Verification items for the finished model (mm, model axes). A direction names the side the tool comes from. Give positions to 0.01 mm unless a question says otherwise; leave off trailing zeros. Write each loop counter-clockwise with the first axis right and the second up, starting at its lowest first coordinate (ties: lowest second). Pieces come first, ordered by that corner, then holes.
from build123d import *

# Parameters (mm, degrees)
SKETCH_1_W             = 38
SKETCH_1_H             = 30
SKETCH_1_R             = 1.65
EXTRUDE_694_DEPTH      = 25
SKETCH_3_W             = 20
SKETCH_3_H             = 30
CUT_EXTRUDE_926_DEPTH  = 15
SKETCH_4_W             = 2.3
SKETCH_4_H             = 15
CUT_EXTRUDE_1406_DEPTH = 55.488530903
FILLET_3_R             = 1
FILLET_4_R             = 2
SKETCH_6_R             = 1.75
CUT_EXTRUDE_2902_DEPTH = 55.488530903
SKETCH_7_R             = 3.5
CUT_EXTRUDE_3145_DEPTH = 10
CUT_EXTRUDE_3527_DEPTH = 3


with BuildPart() as part:
    # Эскиз1 → Extrude 694 (new body)
    with BuildSketch(Plane(origin=(0, 0, 0), x_dir=(1, 0, 0), z_dir=(0, 1, 0))):
        with Locations((19, 15)):
            Rectangle(SKETCH_1_W, SKETCH_1_H)
        with Locations(Location((14.050252532, 24.949747468, 0), (0, 0, 270))):
            Circle(SKETCH_1_R, mode=Mode.SUBTRACT)
        with Locations(Location((23.949747468, 24.949747468, 0), (0, 0, 270))):
            Circle(SKETCH_1_R, mode=Mode.SUBTRACT)
        with Locations(Location((23.949747468, 15.050252532, 0), (0, 0, 270))):
            Circle(SKETCH_1_R, mode=Mode.SUBTRACT)
        with Locations(Location((14.050252532, 15.050252532, 0), (0, 0, 270))):
            Circle(SKETCH_1_R, mode=Mode.SUBTRACT)
    extrude(amount=EXTRUDE_694_DEPTH)

    # Эскиз3 → Cut-Extrude 926 (cut)
    with BuildSketch(Plane(origin=(0, 25, 0), x_dir=(1, 0, 0), z_dir=(0, 1, 0))):
        with Locations((19, 15)):
            Rectangle(SKETCH_3_W, SKETCH_3_H)
    extrude(amount=-CUT_EXTRUDE_926_DEPTH, mode=Mode.SUBTRACT)

    # Эскиз4 → Cut-Extrude 1406 (cut, through all)
    with BuildSketch(Plane.ZY):
        Polygon((-30, 10), (-23, 25), (-30, 25), align=None)
        with Locations((-9.900252532, 17.5)):
            Rectangle(SKETCH_4_W, SKETCH_4_H)
    extrude(amount=-CUT_EXTRUDE_1406_DEPTH, mode=Mode.SUBTRACT)

    # Скругление3
    fillet_3_edges = [part.edges().sort_by_distance(p)[0] for p in [
        (4.5, 25, -11.050252532),
        (33.5, 25, -11.050252532),
        (4.5, 25, -8.750252532),
        (33.5, 25, -8.750252532),
    ]]
    fillet(fillet_3_edges, radius=FILLET_3_R)

    # Скругление4
    fillet_4_edges = [part.edges().sort_by_distance(p)[0] for p in [
        (9, 17.5, 0),
        (19, 10, 0),
        (29, 17.5, 0),
        (38, 0, -15),
        (0, 0, -15),
        (9, 17.5, -26.5),
        (29, 17.5, -26.5),
        (38, 17.5, -26.5),
        (0, 17.5, -26.5),
    ]]
    fillet(fillet_4_edges, radius=FILLET_4_R)

    # Эскиз6 → Cut-Extrude 2902 (cut, through all)
    with BuildSketch(Plane(origin=(0, 0, -30), x_dir=(-1, 0, 0), z_dir=(0, 0, -1))):
        with Locations((-34, 15)):
            Circle(SKETCH_6_R)
        with Locations((-4, 15)):
            Circle(SKETCH_6_R)
    extrude(amount=-CUT_EXTRUDE_2902_DEPTH, mode=Mode.SUBTRACT)

    # Эскиз7 → Cut-Extrude 3145 (cut)
    with BuildSketch(Plane(origin=(0, 0, -30), x_dir=(-1, 0, 0), z_dir=(0, 0, -1))):
        with Locations((-34, 15)):
            Circle(SKETCH_7_R)
        with Locations((-4, 15)):
            Circle(SKETCH_7_R)
    extrude(amount=-CUT_EXTRUDE_3145_DEPTH, mode=Mode.SUBTRACT)

    # Эскиз8 → Cut-Extrude 3527 (cut)
    with BuildSketch(Plane.XY):
        Polygon((7, 13.267949192), (7, 16.732050808), (4, 18.464101615), (1, 16.732050808), (1, 13.267949192), (4, 11.535898385), align=None)
        Polygon((34, 18.464101615), (31, 16.732050808), (31, 13.267949192), (34, 11.535898385), (37, 13.267949192), (37, 16.732050808), align=None)
    extrude(amount=-CUT_EXTRUDE_3527_DEPTH, mode=Mode.SUBTRACT)


solid = part.part
Item 1: Scan lines: line 1 along Z through (x, y) = (13.5, 9); line 2 along X through (y, z) = (11.5, -8.5); line 3 along X through (y, z) = (15, -24.5). Record each from-to range of solid material in increasing order.
Answer key:
line 1: z = -30 to -26.51, -23.39 to -16.61, -13.49 to -0.27
line 2: x = 0 to 9, 29 to 38
line 3: x = 0 to 0.5, 7.5 to 9, 29 to 30.5, 37.5 to 38
Item 2: Sectioned sample at D-D on z = -10. Record the cut outline in (x, y), then the cut area to 3 significant figures.
Answer key:
outline: (0, 2) arc R2 ccw to (2, 0) - (36, 0) arc R2 ccw to (38, 2) - (38, 10) - (0, 10) - close
area: 378 mm2
Item 3: Release check for a two-part mould opening along Y. For faces 5 (the face through (4, 17, -11.05)), 6 (the face through (3, 17, -20)), 7 (the face through (33.465, 21.755, -24.514)), 8 (the face through (35.29, 16.18, -5.92)) record: released by +Y, released by -Y, zero draft, split by the parting line, or undercut.
Answer key:
face 5: zero draft
face 6: undercut
face 7: released by +Y
face 8: undercut
Item 4: Depth check by flat-ended pin: pin 1 (4 mm diameter, centred on x = 34, y = 15, fed in from +Z); pin 2 (3 mm diameter, centred on x = 14.05, z = -24.95, fed in from +Y) (1 decimal); pin 3 (7.5 mm diameter, centred on x = 4.5, y = 16, fed in from -Z); pin 4 (4.5 mm diameter, centred on x = 4, y = 15, fed in from -Z). Enter the tip coordinate at first touch or a pass-through.
Answer key:
pin 1: stops at z = -3
pin 2: passes through
pin 3: stops at z = -28.5
pin 4: stops at z = -20
Item 5: Sectioned sample at B-B on x = 10.5. Record the cut outline in (y, z), then the cut area to 3 significant figures.
Answer key:
outline: (0, -30) - (10, -30) - (10, -2) arc R2 ccw to (8, 0) - (0, 0) - close
area: 299 mm2
Item 6: Sectioned sample at A-A on x = 3. Record the cut outline in (y, z), then the cut area to 3 significant figures.
Answer key:
outline: (0, -30) - (10, -30) - (11.65, -29.23) - (11.65, -20) - (13.56, -20) - (13.56, -11.05) - (10, -11.05) - (10, -8.75) - (13.56, -8.75) - (13.56, -3) - (12.11, -3) - (12.11, 0) - (0, 0) - close; (16.44, -20) - (18.35, -20) - (18.35, -26.1) - (25, -23) - (25, -12.05) arc R1 ccw to (24, -11.05) - (16.44, -11.05) - close; (16.44, -8.75) - (24, -8.75) arc R1 ccw to (25, -7.75) - (25, 0) - (17.89, 0) - (17.89, -3) - (16.44, -3) - close
area: 552 mm2
Item 7: Set-up check for faces 1 (the face through (8.4, 16.38, -0.57)), 2 (the face through (5.5, 12.4, -1.5)), 3 (the face through (29, 18, -17)), 4 (the face through (33.563, 24.715, -8.45)): record each of +Z, -Z, +X, -X, +Y, -Y from which the full face is reachable in a straight line by a thin tool's end or side.
Answer key:
face 1: +Z, +Y
face 2: +Z
face 3: +Z, -Z, +Y
face 4: +X, -X, +Y
Item 8: Sectioned sample at C-C on y = 3.25. Record the cut outline in (x, z).
Answer key:
outline: (0, -30) - (38, -30) - (38, 0) - (0, 0) - close; hole circle Ø3.3 at (14.05, -24.95); hole circle Ø3.3 at (14.05, -15.05); hole circle Ø3.3 at (23.95, -24.95); hole circle Ø3.3 at (23.95, -15.05)
